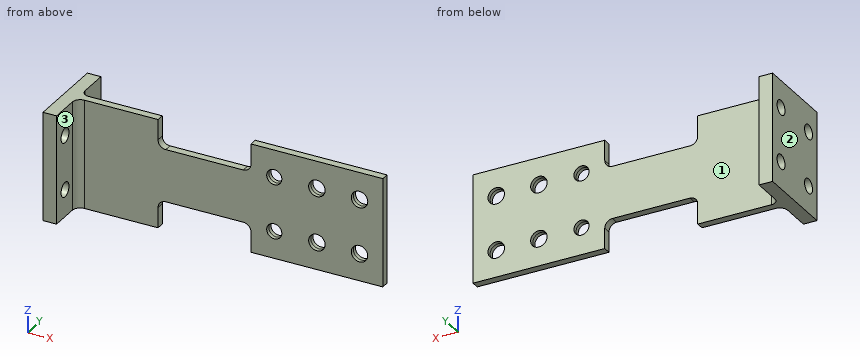
from build123d import *

# Parameters (mm, degrees)
F0_R     = 12.372008059
F0_R_2   = 13.49375
F1_DEPTH = 6.35
F2_DEPTH = 6.35
F3_R     = 11.90625
F4_DEPTH = 22.225
F5_R     = 12.7


with BuildPart() as f1:
    # F0 (on Front) → F1 (new body)
    with BuildSketch(Plane.XZ):
        with BuildLine():
            Line((0, 88.9), (0, 0))
            Line((0, 0), (0, -88.9))
            Line((0, -88.9), (155.575, -88.9))
            Line((155.575, -88.9), (155.575, -55.5625))
            ThreePointArc((155.575, -55.5625), (159.2947438789, -46.5822438789), (168.275, -42.8625))
            Line((168.275, -42.8625), (295.275, -42.8625))
            ThreePointArc((295.275, -42.8625), (304.2552561211, -46.5822438789), (307.975, -55.5625))
            Line((307.975, -55.5625), (307.975, -88.9))
            Line((307.975, -88.9), (523.875, -88.9))
            Line((523.875, -88.9), (523.875, 0))
            Line((523.875, 0), (523.875, 88.9))
            Line((523.875, 88.9), (307.975, 88.9))
            Line((307.975, 88.9), (307.975, 55.5625))
            ThreePointArc((307.975, 55.5625), (304.2552561211, 46.5822438789), (295.275, 42.8625))
            Line((295.275, 42.8625), (168.275, 42.8625))
            ThreePointArc((168.275, 42.8625), (159.2947438789, 46.5822438789), (155.575, 55.5625))
            Line((155.575, 55.5625), (155.575, 88.9))
            Line((155.575, 88.9), (0, 88.9))
        make_face()
        with Locations((346.075, -44.45)):
            Circle(F0_R, mode=Mode.SUBTRACT)
        with Locations((415.925, -44.45)):
            Circle(F0_R_2, mode=Mode.SUBTRACT)
        with Locations((485.775, -44.45)):
            Circle(F0_R_2, mode=Mode.SUBTRACT)
        with Locations((346.075, 44.45)):
            Circle(F0_R, mode=Mode.SUBTRACT)
        with Locations((415.925, 44.45)):
            Circle(F0_R_2, mode=Mode.SUBTRACT)
        with Locations((485.775, 44.45)):
            Circle(F0_R_2, mode=Mode.SUBTRACT)
    extrude(amount=F1_DEPTH)

    # F2 (add): a face of the model
    f2_faces = [f1.faces().sort_by_distance(p)[0] for p in [
        (260.6993813627, 0, 0),
    ]]
    extrude(f2_faces, amount=F2_DEPTH)

    # F3 (on Right) → F4 (join)
    with BuildSketch(Plane.YZ):
        Polygon((66.675, 88.9), (0, 88.9), (-66.675, 88.9), (-66.675, 0), (-66.675, -88.9), (0, -88.9), (66.675, -88.9), (66.675, 0), align=None)
        with Locations((-41.275, -44.45)):
            Circle(F3_R, mode=Mode.SUBTRACT)
        with Locations((41.275, -44.45)):
            Circle(F3_R, mode=Mode.SUBTRACT)
        with Locations((-41.275, 44.45)):
            Circle(F3_R, mode=Mode.SUBTRACT)
        with Locations((41.275, 44.45)):
            Circle(F3_R, mode=Mode.SUBTRACT)
    extrude(amount=F4_DEPTH)

    # F5
    f5_edges = [f1.edges().sort_by_distance(p)[0] for p in [
        (22.225, 6.35, 0),
        (22.225, -6.35, 0),
    ]]
    fillet(f5_edges, radius=F5_R)


solid = f1.part
Read the model definition and answer for the solid it produces. Units are mm, in the model's axes. Face numbers are marked on the shaded views. A direction names the side the tool comes from. Give positions to 0.01 mm unless a question says otherwise; leave off trailing zeros. Write each loop counter-clockwise with the first axis right and the second up, starting at its lowest first coordinate (ties: lowest second). Pieces come first, ordered by that corner, then holes. Notation, with made-up numbers: (54, 85.25) -> (106, 85.25) arc R10 cw to (106, 95.25) -> close; hole circle Ø9 at (-20, 73). An arc over 180 degrees is marked (long way). Answer as a JSON object with one key per item and string values. Group by question number.
1) Each of these flat-tipped pins is pushed along its axis until it touches: P1, Ø6, axis at x = 338, z = -65, coming from the +Y side; P2, Ø24.5, axis at x = 415.925, z = 44.45, coming from the +Y side; P3, Ø10, axis at x = 202.5, y = 0.5, coming from the +Z side; P4, Ø8, axis at x = 298, y = -4.5, coming from the -Z side. Where does it stop, or does it pass through?
2) Find section C-C (z = -25). Write down the section's boundary in (x, y) (3 decimals), and give its area (3 significant figures).
3) Find section D-D (y = -36). Write down the section's boundary in (x, z) (3 decimals), and give its area (3 significant figures).
4) A tool of negligible diameter and unlimited length cuts with its end or side. For the marked faces 1, 2 and 3, from which of +Z, -Z, +X, -X, +Y, -Y can it reach the whole face along a straight path? Write none if from no direction.
5) Consider L1, parallel to X at y = 3, z = 44 (3 decimals); L2, parallel to X at y = 56, z = -23 (3 decimals); L3, parallel to Y at x = 309.5, z = -14. Determine where each line is inside the solid, lowest interval first. Write a range as from..to.
6) Find section B-B (x = 423.5). Write down the section's boundary in (y, z), and give its area (3 significant figures).
7) Find section A-A (z = 72). Write down the section's boundary in (x, y) (3 decimals), and give its area (3 significant figures).
Values follow:
{
 "1": {"P1": "stops at y = 6.35", "P2": "passes through", "P3": "stops at z = 42.86", "P4": "stops at z = -44.79"},
 "2": {"outline": "(0, -66.675) -> (22.225, -66.675) -> (22.225, -19.05) arc R12.7 cw to (34.925, -6.35) -> (523.875, -6.35) -> (523.875, 6.35) -> (34.925, 6.35) arc R12.7 cw to (22.225, 19.05) -> (22.225, 66.675) -> (0, 66.675) -> close", "area": "9,400 mm2"},
 "3": {"outline": "(0, -88.9) -> (22.225, -88.9) -> (22.225, -55.124) -> (0, -55.124) -> close; (0, -33.776) -> (22.225, -33.776) -> (22.225, 33.776) -> (0, 33.776) -> close; (0, 55.124) -> (22.225, 55.124) -> (22.225, 88.9) -> (0, 88.9) -> close", "area": "3,000 mm2"},
 "4": {"face 1": "+Z, -Z, +X, +Y", "face 2": "+Z, -Z, -X, +Y, -Y", "face 3": "+Z, -Z, +X, -Y"},
 "5": {"L1": "x = 0..163.022, 300.528..333.711, 358.439..402.439, 429.411..472.289, 499.261..523.875", "L2": "x = 0..22.225", "L3": "y = -6.35..6.35"},
 "6": {"outline": "(-6.35, -88.9) -> (6.35, -88.9) -> (6.35, -55.62) -> (-6.35, -55.62) -> close; (-6.35, -33.28) -> (6.35, -33.28) -> (6.35, 33.28) -> (-6.35, 33.28) -> close; (-6.35, 55.62) -> (6.35, 55.62) -> (6.35, 88.9) -> (-6.35, 88.9) -> close", "area": "1,690 mm2"},
 "7": {"outline": "(0, -66.675) -> (22.225, -66.675) -> (22.225, -19.05) arc R12.7 cw to (34.925, -6.35) -> (155.575, -6.35) -> (155.575, 6.35) -> (34.925, 6.35) arc R12.7 cw to (22.225, 19.05) -> (22.225, 66.675) -> (0, 66.675) -> close; (307.975, -6.35) -> (523.875, -6.35) -> (523.875, 6.35) -> (307.975, 6.35) -> close", "area": "7,470 mm2"}
}
